For this review, use the dimensioned drawing (mm, ordinates from the lowest corner) and the shaded views. A direction names the side the tool comes from. Give positions to 0.01 mm unless a question says otherwise; leave off trailing zeros. Loops run counter-clockwise (first coordinate to the right, second up) from the corner with the lowest first, then second, coordinate; pieces in that order, holes last. Notation, with made-up numbers: M -25.5,-4 L 11.5,-4 A29 cw 11.5,29 Z; hole C -34,73.25 d4. An arc over 180 degrees is marked long. Use CSV: the item, a comma, the result in double quotes.
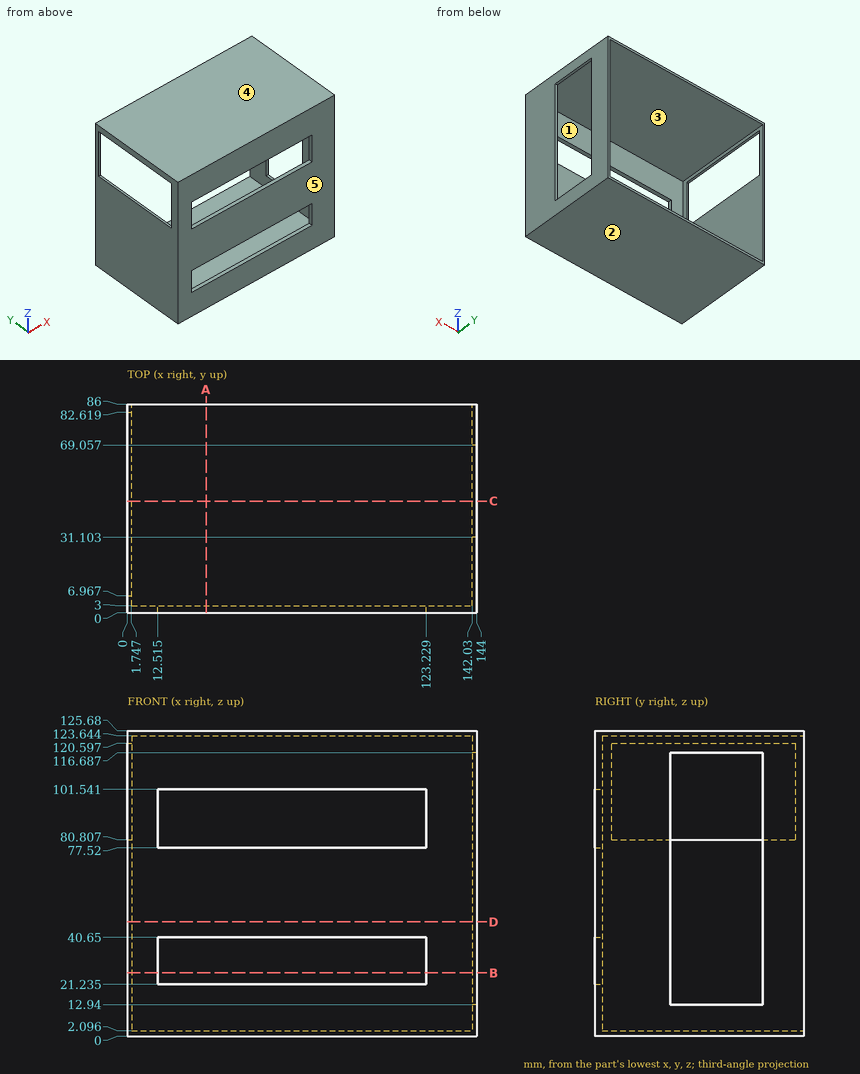
(1) The part is to be moulded in two halves that separate along Z. For the marked faces 3, 4 and 5, say which applies: released by +Z, released by -Z, zero draft, split by the parting line, or undercut.
A:
face 3,"undercut"
face 4,"released by +Z"
face 5,"zero draft"
(2) We need section D-D on z = 47. State the section outline as (x, y) points.
A:
outline,"M 0,0 L 144,0 L 144,31.1 L 142.03,31.1 L 142.03,3 L 1.75,3 L 1.75,86 L 0,86 Z; M 142.03,69.06 L 144,69.06 L 144,86 L 142.03,86 Z"
(3) We need section B-B on z = 26. State the section outline as (x, y) points (1 decimal).
A:
outline,"M 0,0 L 12.5,0 L 12.5,3 L 1.7,3 L 1.7,86 L 0,86 Z; M 123.2,0 L 144,0 L 144,31.1 L 142,31.1 L 142,3 L 123.2,3 Z; M 142,69.1 L 144,69.1 L 144,86 L 142,86 Z"
(4) Machinability: for the marked faces 1 and 2, which of the approach directions +Z, -Z, +X, -X, +Y, -Y give a long, thin tool a straight path to every point of the face, cutting with its end or side? Answer none if there is none.
A:
face 1,"+Y"
face 2,"-Z, +X, -X, +Y, -Y"
(5) We need section C-C on y = 46. State the section outline as (x, z) points (1 decimal).
A:
outline,"M 0,0 L 144,0 L 144,12.9 L 142,12.9 L 142,2.1 L 1.7,2.1 L 1.7,80.8 L 0,80.8 Z; M 0,120.6 L 1.7,120.6 L 1.7,123.6 L 142,123.6 L 142,116.7 L 144,116.7 L 144,125.7 L 0,125.7 Z"
(6) We need section A-A on x = 32.5. Count the separate pieces of the cut face and the enclosed holes in it.
A:
separate pieces,"3"
enclosed holes,"0"
(7) Wall thickness on line 1 along Z through (x, y) = (51, 69) (1 decimal); line 2 along X through (y, z) = (14.5, 38); line 3 along Y through (x, z) = (70, 52): over which ranges is each line inside the solid? List them lowest first. Write a range as [from, to].
A:
line 1,"[0, 2.1], [123.6, 125.7]"
line 2,"[0, 1.75], [142.03, 144]"
line 3,"[0, 3]"
(8) Clearance check with flat-ended pins moving along their axes: P1, Ø12, axis at x = 92, z = 76, coming from the +Y side; P2, Ø12, axis at x = 80.5, z = 27.5, coming from the +Y side. State where each tip first meets the part, or that it passes through.
A:
P1,"y = 3"
P2,"through"
